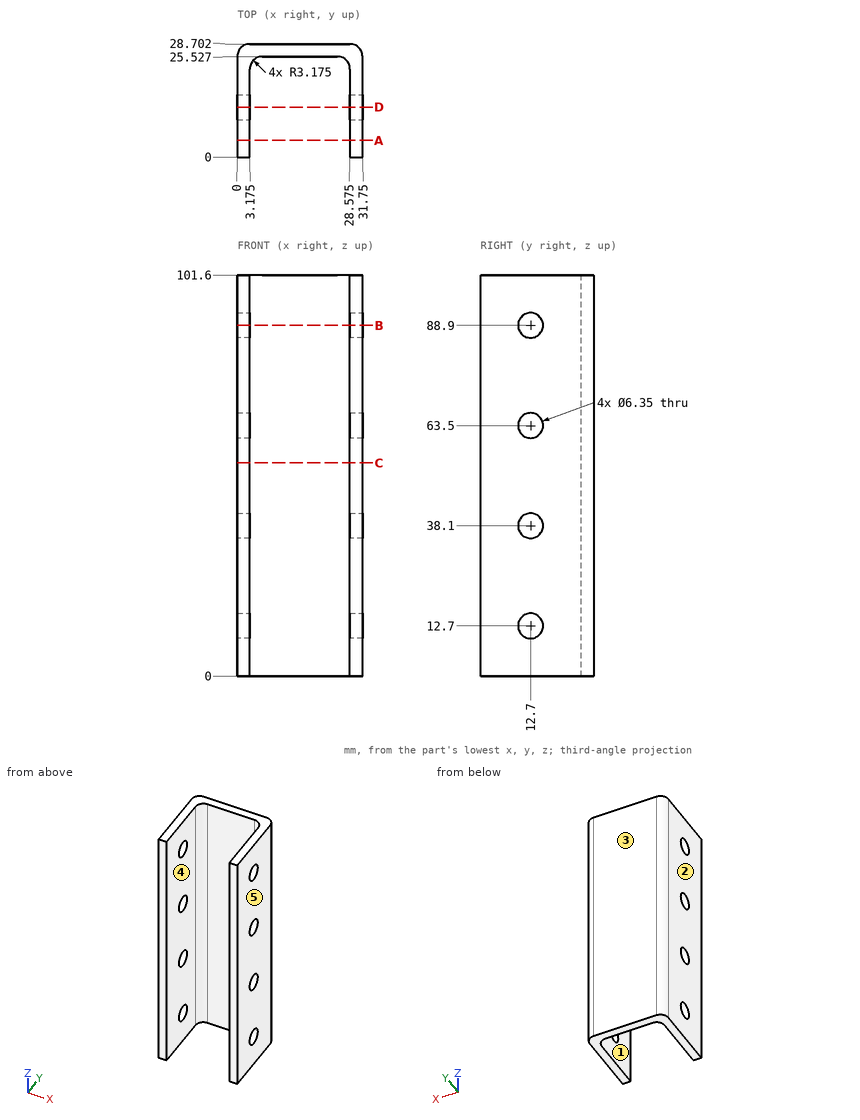
Print and shaded views of the part. All mm, measured from the part's lowest x, y and z. A direction names the side the tool comes from. Coordinates: 2 decimals unless noted, no trailing zeros. Write each loop counter-clockwise with the first axis right and the second up, starting at its lowest first coordinate (ties: lowest second). Pieces come first, ordered by that corner, then holes. Notation, with made-up numbers: (-7, 17.25) -> (23, 17.25) arc R15 ccw to (23, 36.25) -> close; hole circle Ø8 at (83.25, 77.25). An arc over 180 degrees is marked (long way). Use CSV: the item, a comma, the result in double quotes. Start each with the question number.
Q1. 3-axis set-ups, long thin cutter, end or side, ignore diameter. For the marked faces 1 and 2: which of +Z, -Z, +X, -X, +Y, -Y reach the whole face in a straight line?
Q2. Flat gauge pins, fed straight in: pin 1 Ø3 at (x, z) = (14.5, 74.5) entering from -Y; pin 2 Ø15 at (x, z) = (20.5, 33.5) entering from -Y; pin 3 Ø10 at (y, z) = (12.7, 12.7) entering from +X; pin 4 Ø12 at (x, z) = (21, 12.5) entering from -Y. Where does each tip first touch, or does it go through?
Q3. Drill centre lines: probe 1 along X at (y, z) = (20, 92) (3 decimals); probe 2 along X at (y, z) = (25, 54); probe 3 along Y at (x, z) = (1.4, 63.5) (3 decimals). Where is each one in solid material? Low to high.
Q4. Cut at A-A, the plane y = 4.25. List the corners of the cut face in (x, z) (3 decimals).
Q5. Pull direction X, two halves, no side cores. Call the marked faces 3, 4 and 5: released by +X, released by -X, zero draft, split by the parting line, or undercut.
Q6. Cut at C-C, the plane z = 54. List the corners of the cut face in (x, y) (3 decimals), then the cut area to 3 significant figures.
Q7. Cut at D-D, the plane y = 12.7. State how many separate pieces and enclosed holes the cut face has, then the cut area to 3 significant figures.
Q8. Cut at B-B, the plane z = 88.9. List the corners of the cut face in (x, y) (3 decimals).
Checked values:
1,face 1,"+Z, -Z, -Y"
1,face 2,"+Z, -Z, -X, +Y, -Y"
2,pin 1,"stops at y = 25.53"
2,pin 2,"stops at y = 24.17"
2,pin 3,"stops at x = 31.75"
2,pin 4,"stops at y = 25.09"
3,probe 1,"x = 0 to 3.175, 28.575 to 31.75"
3,probe 2,"x = 0 to 4.6, 27.15 to 31.75"
3,probe 3,"y = 0 to 9.525, 15.875 to 28.159"
4,outline,"(0, 0) -> (3.175, 0) -> (3.175, 101.6) -> (0, 101.6) -> close; (28.575, 0) -> (31.75, 0) -> (31.75, 101.6) -> (28.575, 101.6) -> close"
5,face 3,"zero draft"
5,face 4,"undercut"
5,face 5,"released by +X"
6,outline,"(0, 0) -> (3.175, 0) -> (3.175, 22.352) arc R3.175 cw to (6.35, 25.527) -> (25.4, 25.527) arc R3.175 cw to (28.575, 22.352) -> (28.575, 0) -> (31.75, 0) -> (31.75, 25.527) arc R3.175 ccw to (28.575, 28.702) -> (3.175, 28.702) arc R3.175 ccw to (0, 25.527) -> close"
6,area,"263 mm²"
7,separate pieces,"10"
7,enclosed holes,"0"
7,area,"484 mm²"
8,outline,"(0, 0) -> (3.175, 0) -> (3.175, 9.525) -> (0, 9.525) -> close; (0, 15.875) -> (3.175, 15.875) -> (3.175, 22.352) arc R3.175 cw to (6.35, 25.527) -> (25.4, 25.527) arc R3.175 cw to (28.575, 22.352) -> (28.575, 15.875) -> (31.75, 15.875) -> (31.75, 25.527) arc R3.175 ccw to (28.575, 28.702) -> (3.175, 28.702) arc R3.175 ccw to (0, 25.527) -> close; (28.575, 0) -> (31.75, 0) -> (31.75, 9.525) -> (28.575, 9.525) -> close"
